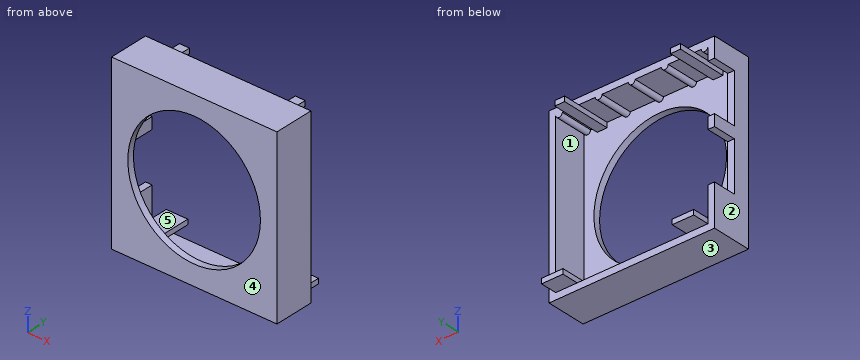
```python
from build123d import *

# Parameters (mm, degrees)
SKETCH2_W           = 50
SKETCH2_H           = 52
BOSS_EXTRUDE1_DEPTH = 12
SKETCH5_W           = 46
SKETCH5_H           = 48
CUT_EXTRUDE1_DEPTH  = 10
SKETCH7_W           = 2
SKETCH7_H           = 15
CUT_EXTRUDE2_DEPTH  = 7
SKETCH10_R          = 1
BOSS_EXTRUDE2_DEPTH = 10
SKETCH11_W          = 3
SKETCH11_H          = 1.5
SKETCH11_W_2        = 6.5
SKETCH11_H_2        = 1.499602214
BOSS_EXTRUDE3_DEPTH = 15
SKETCH12_R          = 20.034029424
CUT_EXTRUDE4_DEPTH  = 15


with BuildPart() as part:
    # Sketch2 → Boss-Extrude1 (new body)
    with BuildSketch(Plane(origin=(0, 0, 0), x_dir=(1, 0, 0), z_dir=(0, 1, 0))):
        with Locations((25, 26)):
            Rectangle(SKETCH2_W, SKETCH2_H)
    extrude(amount=BOSS_EXTRUDE1_DEPTH)

    # Sketch5 → Cut-Extrude1 (cut)
    with BuildSketch(Plane(origin=(0, 12, 0), x_dir=(1, 0, 0), z_dir=(0, 1, 0))):
        with Locations((25, 26)):
            Rectangle(SKETCH5_W, SKETCH5_H)
    extrude(amount=-CUT_EXTRUDE1_DEPTH, mode=Mode.SUBTRACT)

    # Sketch7 → Cut-Extrude2 (cut)
    with BuildSketch(Plane(origin=(0, 12, 0), x_dir=(1, 0, 0), z_dir=(0, 1, 0))):
        with Locations((1, 32)):
            Rectangle(SKETCH7_W, SKETCH7_H)
        with Locations((1, 13.5)):
            Rectangle(SKETCH7_W, SKETCH7_H)
    extrude(amount=-CUT_EXTRUDE2_DEPTH, mode=Mode.SUBTRACT)

    # Sketch10 → Boss-Extrude2 (add)
    with BuildSketch(Plane(origin=(0, 2, 0), x_dir=(1, 0, 0), z_dir=(0, 1, 0))):
        with Locations((25, 2)):
            Circle(SKETCH10_R)
        with Locations((35, 2)):
            Circle(SKETCH10_R)
        with Locations((15, 2)):
            Circle(SKETCH10_R)
        with Locations((3, 2)):
            Circle(SKETCH10_R)
        with Locations((47, 2)):
            Circle(SKETCH10_R)
    extrude(amount=BOSS_EXTRUDE2_DEPTH)

    # Sketch11 → Boss-Extrude3 (add)
    with BuildSketch(Plane(origin=(0, 2, 0), x_dir=(1, 0, 0), z_dir=(0, 1, 0))):
        with Locations((7.5, 2.75)):
            Rectangle(SKETCH11_W, SKETCH11_H)
        with Locations((42.5, 2.75)):
            Rectangle(SKETCH11_W, SKETCH11_H)
        with Locations((5.25, 49.250198893)):
            Rectangle(SKETCH11_W_2, SKETCH11_H_2)
        with Locations((44.75, 49.250198893)):
            Rectangle(SKETCH11_W_2, SKETCH11_H_2)
    extrude(amount=BOSS_EXTRUDE3_DEPTH)

    # Sketch12 → Cut-Extrude4 (cut)
    with BuildSketch(Plane(origin=(0, 2, 0), x_dir=(1, 0, 0), z_dir=(0, 1, 0))):
        with Locations(Location((24.959746772, 25.897804051, 0), (0, 0, 270))):
            Circle(SKETCH12_R)
    extrude(amount=-CUT_EXTRUDE4_DEPTH, mode=Mode.SUBTRACT)


solid = part.part
```
The model under review builds one solid part; all positions refer to its coordinate system, in mm. Face numbers are marked on the shaded views. A direction names the side the tool comes from. Round coordinates to 2 decimals unless told otherwise and drop trailing zeros. Loops run counter-clockwise (first coordinate to the right, second up) from the corner with the lowest first, then second, coordinate; pieces in that order, holes last.
1) Clearance check with flat-ended pins moving along their axes: P1, Ø1.5, axis at x = 8, y = 14.5, coming from the +Z side; P2, Ø4, axis at x = 6, y = 15.5, coming from the -Z side; P3, Ø12, axis at x = 39, z = -9.5, coming from the +Y side. State where each tip first meets the part, or that it passes through.
Values follow:
P1: stops at z = -2
P2: stops at z = -50
P3: stops at y = 2
2) Consider section B-B on x = 43. State the section outline as (y, z) points.
Values follow:
outline: (0, -52) - (12, -52) - (12, -50) - (17, -50) - (17, -48.5) - (2, -48.5) - (2, -34.61) - (0, -34.61) - close; (0, -17.19) - (2, -17.19) - (2, -3.5) - (17, -3.5) - (17, -2) - (12, -2) - (12, 0) - (0, 0) - close
3) Wall thickness on line 1 along X through (y, z) = (11.75, -47); line 2 along Z through (x, y) = (15, 11); line 3 along Z through (x, y) = (42, 3.25): over which ranges is each line inside the solid? List them lowest first.
Values follow:
line 1: x = 0 to 2, 48 to 50
line 2: z = -52 to -50, -3 to 0
line 3: z = -52 to -48.5, -3.5 to 0
4) Consider section C-C on z = -38.5. State the section outline as (x, y) points, then the cut area to 3 significant figures.
Values follow:
outline: (0, 0) - (9.39, 0) - (9.39, 2) - (2, 2) - (2, 5) - (0, 5) - close; (40.53, 0) - (50, 0) - (50, 12) - (48, 12) - (48, 2) - (40.53, 2) - close
area: 63.7 mm2
5) Consider section A-A on y = 13.5. State the section outline as (x, z) points.
Values follow:
outline: (2, -50) - (8.5, -50) - (8.5, -48.5) - (2, -48.5) - close; (6, -3.5) - (9, -3.5) - (9, -2) - (6, -2) - close; (41, -3.5) - (44, -3.5) - (44, -2) - (41, -2) - close; (41.5, -50) - (48, -50) - (48, -48.5) - (41.5, -48.5) - close
6) Consider section D-D on z = -47.5. State the section outline as (x, y) points.
Values follow:
outline: (0, 0) - (50, 0) - (50, 12) - (48, 12) - (48, 2) - (2, 2) - (2, 12) - (0, 12) - close
7) The part is to be moulded in two halves that separate along X. For the marked faces 1, 2 and 3, say which applies: pulls with the +X half, pulls with the -X half, needs draft (parallel to the pull), parting line crosses it, or undercut.
Values follow:
face 1: undercut
face 2: pulls with the -X half
face 3: needs draft
8) Tool access review of the marked faces 4 and 5: name each direction out of +Z, -Z, +X, -X, +Y, -Y from which nothing blocks a thin tool from reaching the whole face with its end or side.
Values follow:
face 4: +Z, -Z, +X, -X, -Y
face 5: +Y
